For this review, use the dimensioned drawing (mm, ordinates from the lowest corner) and the shaded views. A direction names the side the tool comes from. Coordinates: 2 decimals unless noted, no trailing zeros. Write each loop counter-clockwise with the first axis right and the second up, starting at its lowest first coordinate (ties: lowest second). Pieces come first, ordered by that corner, then holes.
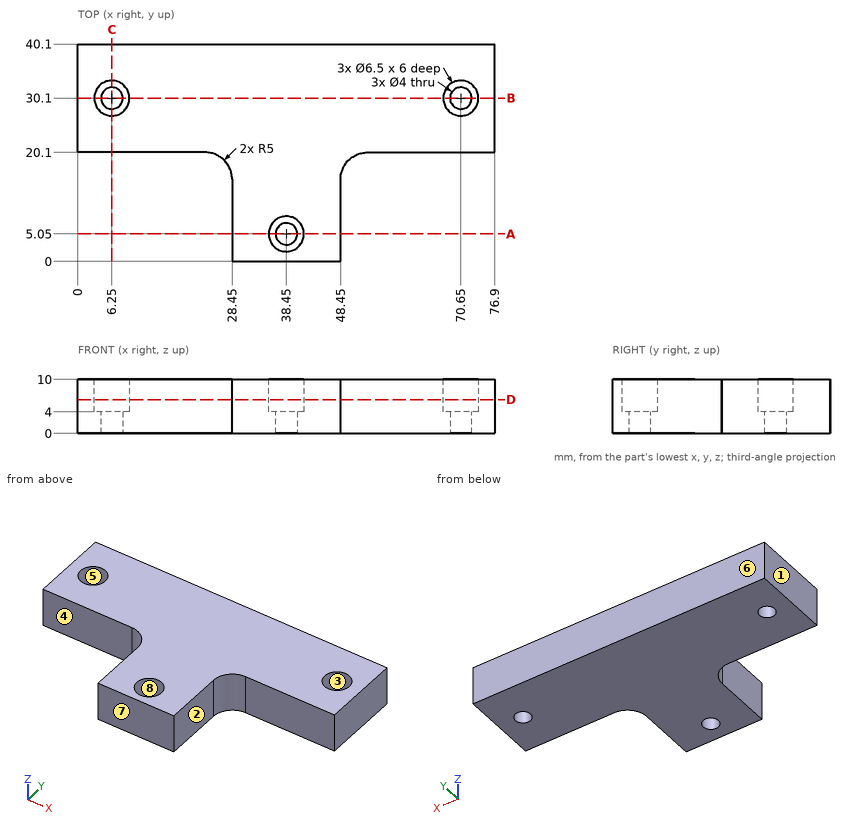
Item 1: Take a section at B-B, the plane y = 30.1. Write out the cut boundary in (x, z).
Solved:
outline: (0, 0) - (4.25, 0) - (4.25, 4) - (3, 4) - (3, 10) - (0, 10) - close; (8.25, 0) - (68.65, 0) - (68.65, 4) - (67.4, 4) - (67.4, 10) - (9.5, 10) - (9.5, 4) - (8.25, 4) - close; (72.65, 0) - (76.9, 0) - (76.9, 10) - (73.9, 10) - (73.9, 4) - (72.65, 4) - close
Item 2: For pin 1 (3 mm diameter, centred on x = 64, z = 6, fed in from -Y); pin 2 (6 mm diameter, centred on y = 4.5, z = 2, fed in from -X); pin 3 (6.5 mm diameter, centred on x = 38.45, y = 5.05, fed in from -Z), all flat-tipped, find the tip position at first contact; note any pin that passes through.
Solved:
pin 1: stops at y = 20.1
pin 2: stops at x = 28.45
pin 3: stops at z = 0
Item 3: To check wall thickness, follow line 1 along Y through (x, z) = (6.25, 1.2); line 2 along Y through (x, z) = (70.65, 6.05); line 3 along Y through (x, z) = (65.5, 2). State the ranges of each line that lie inside material, in increasing order.
Solved:
line 1: y = 20.1 to 28.1, 32.1 to 40.1
line 2: y = 20.1 to 26.85, 33.35 to 40.1
line 3: y = 20.1 to 40.1
Item 4: Mouldability with a two-part tool opening along Y and no side actions: class the marked faces 5, 6, 7 and 8 as pulls with the +Y half, pulls with the -Y half, needs draft (parallel to the pull), parting line crosses it, or undercut.
Solved:
face 5: undercut
face 6: pulls with the +Y half
face 7: pulls with the -Y half
face 8: undercut
Item 5: Take a section at D-D, the plane z = 6.25. Write out the cut boundary in (x, y).
Solved:
outline: (0, 20.1) - (23.45, 20.1) arc R5 cw to (28.45, 15.1) - (28.45, 0) - (48.45, 0) - (48.45, 15.1) arc R5 cw to (53.45, 20.1) - (76.9, 20.1) - (76.9, 40.1) - (0, 40.1) - close; hole circle Ø6.5 at (6.25, 30.1); hole circle Ø6.5 at (38.45, 5.05); hole circle Ø6.5 at (70.65, 30.1)
Item 6: Machinability: for the marked faces 1, 2, 3 and 4, which of the approach directions +Z, -Z, +X, -X, +Y, -Y give a long, thin tool a straight path to every point of the face, cutting with its end or side? Answer none if there is none.
Solved:
face 1: +Z, -Z, -X, +Y, -Y
face 2: +Z, -Z, +X, -Y
face 3: +Z
face 4: +Z, -Z, -X, -Y
Item 7: Take a section at C-C, the plane x = 6.25. Write out the cut boundary in (y, z).
Solved:
outline: (20.1, 0) - (28.1, 0) - (28.1, 4) - (26.85, 4) - (26.85, 10) - (20.1, 10) - close; (32.1, 0) - (40.1, 0) - (40.1, 10) - (33.35, 10) - (33.35, 4) - (32.1, 4) - close
Item 8: Take a section at A-A, the plane y = 5.05. Write out the cut boundary in (x, z).
Solved:
outline: (28.45, 0) - (36.45, 0) - (36.45, 4) - (35.2, 4) - (35.2, 10) - (28.45, 10) - close; (40.45, 0) - (48.45, 0) - (48.45, 10) - (41.7, 10) - (41.7, 4) - (40.45, 4) - close
